Read the model definition and answer for the solid it produces. Units are mm, in the model's axes. Coordinates: 2 decimals unless noted, no trailing zeros. Order: outer loops, then holes, each group sorted by start corner. A loop starts at its lowest first (then second) coordinate and runs counter-clockwise, first axis right, second up. Notation, with made-up numbers: (72.25, 42) -> (109.25, 42) arc R26 cw to (109.25, 73) -> close; hole circle Ø4 at (66.25, 4.5). An arc over 180 degrees is marked (long way). Answer as a JSON object with one key per item and string values. Group by question number.
1) Consider L1, parallel to Y at x = 1.4, z = -347; L2, parallel to Y at x = 1.1, z = -13.5; L3, parallel to Z at x = 1.45, y = -0.75. Determine where each line is inside the solid, lowest interval first.
2) Section B-B on x = 2 is taken. Determine the outline of the cut face in (y, z).
3) Given pin 1 (1 mm diameter, centred on x = 1, y = 3.5, fed in from +Z), flat-ended and moving along its own axis, determine where the tip first touches the part or whether it passes through.
4) Section A-A on y = 1.5 is taken. Determine the outline of the cut face in (x, z).
from build123d import *

# Parameters (mm, degrees)
SKETCH_1_R      = 1.5
EXTRUDE_1_DEPTH = 3


with BuildPart() as part:
    # 草图1 → 凸台-拉伸1 (new body)
    with BuildSketch(Plane(origin=(0, 0, 0), x_dir=(0, 0, -1), z_dir=(1, 0, 0))):
        with BuildLine():
            Line((0, 5), (394, 5))
            ThreePointArc((394, 5), (397.5, 1.5), (394, -2))
            Line((394, -2), (0, -2))
            ThreePointArc((0, -2), (-3.5, 1.5), (0, 5))
        make_face()
        with Locations((14, 1.5)):
            Circle(SKETCH_1_R, mode=Mode.SUBTRACT)
        with Locations((380, 1.5)):
            Circle(SKETCH_1_R, mode=Mode.SUBTRACT)
        with Locations((47, 1.5)):
            Circle(SKETCH_1_R, mode=Mode.SUBTRACT)
        with Locations((347, 1.5)):
            Circle(SKETCH_1_R, mode=Mode.SUBTRACT)
        with BuildLine():
            ThreePointArc((0, 3), (-1.5, 1.5), (0, 0))
            ThreePointArc((0, 0), (1.5, 1.5), (0, 3))
        make_face(mode=Mode.SUBTRACT)
        with BuildLine():
            ThreePointArc((394, 3), (395.5, 1.5), (394, 0))
            ThreePointArc((394, 0), (392.5, 1.5), (394, 3))
        make_face(mode=Mode.SUBTRACT)
    extrude(amount=EXTRUDE_1_DEPTH)


solid = part.part
Worked answers:
{
 "1": {"L1": "y = -2 to 0, 3 to 5", "L2": "y = -2 to 0.09, 2.91 to 5", "L3": "z = -396.68 to 2.68"},
 "2": {"outline": "(-2, -394) arc R3.5 ccw to (5, -394) -> (5, 0) arc R3.5 ccw to (-2, 0) -> close; hole circle Ø3 at (1.5, -394); hole circle Ø3 at (1.5, -380); hole circle Ø3 at (1.5, -347); hole circle Ø3 at (1.5, -47); hole circle Ø3 at (1.5, -14); hole circle Ø3 at (1.5, 0)"},
 "3": {"pin 1": "stops at z = 3.16"},
 "4": {"outline": "(0, -397.5) -> (3, -397.5) -> (3, -395.5) -> (0, -395.5) -> close; (0, -392.5) -> (3, -392.5) -> (3, -381.5) -> (0, -381.5) -> close; (0, -378.5) -> (3, -378.5) -> (3, -348.5) -> (0, -348.5) -> close; (0, -345.5) -> (3, -345.5) -> (3, -48.5) -> (0, -48.5) -> close; (0, -45.5) -> (3, -45.5) -> (3, -15.5) -> (0, -15.5) -> close; (0, -12.5) -> (3, -12.5) -> (3, -1.5) -> (0, -1.5) -> close; (0, 1.5) -> (3, 1.5) -> (3, 3.5) -> (0, 3.5) -> close"}
}
